Check sheet for the modelled part. Datum: model origin and axes. Units: mm. A direction names the side the tool comes from. Give positions to 0.01 mm unless a question says otherwise; leave off trailing zeros. Loops run counter-clockwise (first coordinate to the right, second up) from the corner with the lowest first, then second, coordinate; pieces in that order, holes last. Notation, with made-up numbers: M -15,11 L 13,11 A13 ccw 13,36 Z; hole C -21,46 d6. An arc over 180 degrees is marked long. Write each question's results on one line, items separated by ' | '. Start each with the question number.
1. Draft check along Z on faces 6 (the cylindrical face through (-19.76, -3.8, -7.67)), 7 (the flat face through (-1, 1, -34)), 8 (the flat face through (37.5, 1, 0)). Enter one of: pulls with the +Z half, pulls with the -Z half, needs draft (parallel to the pull), parting line crosses it, or undercut.
2. Material ranges on line 1 along X through (y, z) = (1.25, 27.5); line 2 along Y through (x, z) = (-1, 26.5); line 3 along Y through (x, z) = (-30.5, -3.5), recorded low to high.
3. Sectioned sample at C-C on x = -11. Record the cut outline in (y, z), and give its area (3 significant figures).
4. Sectioned sample at D-D on y = -2.25. Record the cut outline in (x, z), and give its area (3 significant figures).
5. Tool access check on faces 1 (the cylindrical face through (-18.62, -4.78, 0.39)), 2 (the flat face through (-22, -8, -8)), 3 (the flat face through (-27.5, 5, 0)), 4 (the flat face through (-33, 5, -11)), 5 (the flat face through (-33, 5, 11)). Record the directions out of +Z, -Z, +X, -X, +Y, -Y that give a thin tool (end or side, any length) a straight path to the whole face; none if there is none.
6. Go/stop test with flat-tipped pins: pin 1 (1.8 mm diameter, centred on x = 31.81, z = 28.58, fed in from -Y); pin 2 (4 mm diameter, centred on y = 4.5, z = 10, fed in from +X); pin 3 (5 mm diameter, centred on x = 31.81, z = -28.58, fed in from -Y); pin 4 (5 mm diameter, centred on x = -33.5, y = 5, fed in from +Z). Record where each tip stops, or that it passes through.
7. Sectioned sample at B-B on z = 0. Record the cut outline in (x, y), and give its area (3 significant figures).
8. Sectioned sample at A-A on z = -29. Record the cut outline in (x, y), and give its area (3 significant figures).
```python
from build123d import *

# Parameters (mm, degrees)
SKETCH1_W           = 75
SKETCH1_H           = 68
SKETCH1_R           = 1.5
BOSS_EXTRUDE1_DEPTH = 2
SKETCH2_R           = 3
BOSS_EXTRUDE2_DEPTH = 10
SKETCH3_R           = 2
BOSS_EXTRUDE3_DEPTH = 8
FILLET1_R           = 0.3
SKETCH4_W           = 10
SKETCH4_H           = 22
BOSS_EXTRUDE4_DEPTH = 6


with BuildPart() as part:
    # Sketch1 → Boss-Extrude1 (new body)
    with BuildSketch(Plane(origin=(0, 0, 0), x_dir=(1, 0, 0), z_dir=(0, 1, 0))):
        Rectangle(SKETCH1_W, SKETCH1_H)
        with Locations(Location((31.8135, 28.575, 0), (0, 0, 270))):
            Circle(SKETCH1_R, mode=Mode.SUBTRACT)
        with Locations(Location((31.8135, -28.575, 0), (0, 0, 270))):
            Circle(SKETCH1_R, mode=Mode.SUBTRACT)
        with Locations(Location((-31.6865, 28.575, 0), (0, 0, 270))):
            Circle(SKETCH1_R, mode=Mode.SUBTRACT)
        with Locations(Location((-31.6865, -28.575, 0), (0, 0, 270))):
            Circle(SKETCH1_R, mode=Mode.SUBTRACT)
    extrude(amount=BOSS_EXTRUDE1_DEPTH)

    # Sketch2 → Boss-Extrude2 (add)
    with BuildSketch(Plane.XZ):
        with Locations(Location((-21.592923404, 0, 0), (0, 0, 270))):
            Circle(SKETCH2_R)
    extrude(amount=BOSS_EXTRUDE2_DEPTH)

    # Sketch3 → Boss-Extrude3 (add)
    with BuildSketch(Plane.XZ):
        with Locations(Location((-21.743922868, -7.927471879, 0), (0, 0, 270))):
            Circle(SKETCH3_R)
    extrude(amount=BOSS_EXTRUDE3_DEPTH)

    # Fillet1
    fillet1_edges = [part.edges().sort_by_distance(p)[0] for p in [
        (-21.592923404, -10, 3),
        (-21.743922868, -8, -5.927471879),
    ]]
    fillet(fillet1_edges, radius=FILLET1_R)

    # Sketch4 → Boss-Extrude4 (add)
    with BuildSketch(Plane(origin=(0, 2, 0), x_dir=(1, 0, 0), z_dir=(0, 1, 0))):
        with Locations((-32.5, 0)):
            Rectangle(SKETCH4_W, SKETCH4_H)
    extrude(amount=BOSS_EXTRUDE4_DEPTH)


solid = part.part
```
Output values:
1) face 6: undercut | face 7: pulls with the -Z half | face 8: needs draft
2) line 1: -37.5 to -32.73, -30.64 to 30.77, 32.86 to 37.5 | line 2: 0 to 2 | line 3: 0 to 8
3) outline: M 0,-34 L 2,-34 L 2,34 L 0,34 Z | area: 136 mm2
4) outline: C -21.59,0 d6; C -21.74,-7.93 d4 | area: 40.8 mm2
5) face 1: -Y | face 2: -Z, +X, -X, -Y | face 3: +Z, -Z, +X, +Y | face 4: -Z, +X, -X, +Y | face 5: +Z, +X, -X, +Y
6) pin 1: through | pin 2: x = -27.5 | pin 3: y = 0 | pin 4: z = 11
7) outline: M -37.5,0 L -24.59,0 L -24.59,-9.7 A0.3 ccw -24.29,-10 L -18.89,-10 A0.3 ccw -18.59,-9.7 L -18.59,0 L 37.5,0 L 37.5,2 L -27.5,2 L -27.5,8 L -37.5,8 Z | area: 270 mm2
8) outline: M -37.5,0 L -33.13,0 L -33.13,2 L -37.5,2 Z; M -30.25,0 L 30.37,0 L 30.37,2 L -30.25,2 Z; M 33.25,0 L 37.5,0 L 37.5,2 L 33.25,2 Z | area: 138 mm2
